```python
from build123d import *

# Parameters (mm, degrees)
SKETCH_1_R      = 5
EXTRUDE_1_DEPTH = 60
SKETCH_2_R      = 3.5
EXTRUDE_2_DEPTH = 2
EXTRUDE_START   = 2
SKETCH_3_R      = 3.5
EXTRUDE_3_DEPTH = 2
EXTRUDE_START_2 = 124
SKETCH_4_R      = 5
EXTRUDE_4_DEPTH = 124
SKETCH_5_R      = 5
EXTRUDE_5_DEPTH = 124
SKETCH_6_R      = 3.5
EXTRUDE_6_DEPTH = 2
SKETCH_7_R      = 5
EXTRUDE_7_DEPTH = 10
SKETCH_8_R      = 3.5
EXTRUDE_8_DEPTH = 2
EXTRUDE_START_3 = 10
SKETCH_9_R      = 5
EXTRUDE_9_DEPTH = 10


with BuildPart() as part:
    # 草图1 → 凸台-拉伸1 (new body)
    with BuildSketch(Plane.XY):
        Circle(SKETCH_1_R)
    extrude(amount=EXTRUDE_1_DEPTH)

    # 草图2 → 凸台-拉伸2 (add)
    with BuildSketch(Plane.XY.offset(60)):
        Circle(SKETCH_2_R)
    extrude(amount=EXTRUDE_2_DEPTH)

    # 草图3 → 凸台-拉伸3 (add)
    with BuildSketch(Plane(origin=(0, 0, 0), x_dir=(-1, 0, 0), z_dir=(0, 0, -1)).offset(EXTRUDE_START)):
        with Locations(Location((0, 0, 0), (0, 0, 180))):
            Circle(SKETCH_3_R)
    extrude(amount=-EXTRUDE_3_DEPTH)

    # 草图4 → 凸台-拉伸4 (add)
    with BuildSketch(Plane(origin=(0, 0, -2), x_dir=(-1, 0, 0), z_dir=(0, 0, -1)).offset(EXTRUDE_START_2)):
        with Locations(Location((0, 0, 0), (0, 0, 180))):
            Circle(SKETCH_4_R)
    extrude(amount=-EXTRUDE_4_DEPTH)

    # 草图5 → 凸台-拉伸5 (add)
    with BuildSketch(Plane.XY.offset(62)):
        Circle(SKETCH_5_R)
    extrude(amount=EXTRUDE_5_DEPTH)

    # 草图6 → 凸台-拉伸6 (add)
    with BuildSketch(Plane.XY.offset(186)):
        Circle(SKETCH_6_R)
    extrude(amount=EXTRUDE_6_DEPTH)

    # 草图7 → 凸台-拉伸7 (add)
    with BuildSketch(Plane.XY.offset(188)):
        Circle(SKETCH_7_R)
    extrude(amount=EXTRUDE_7_DEPTH)

    # 草图8 → 凸台-拉伸8 (add)
    with BuildSketch(Plane(origin=(0, 0, -126), x_dir=(-1, 0, 0), z_dir=(0, 0, -1)).offset(EXTRUDE_START)):
        with Locations(Location((0, 0, 0), (0, 0, 180))):
            Circle(SKETCH_8_R)
    extrude(amount=-EXTRUDE_8_DEPTH)

    # 草图9 → 凸台-拉伸9 (add)
    with BuildSketch(Plane(origin=(0, 0, -128), x_dir=(-1, 0, 0), z_dir=(0, 0, -1)).offset(EXTRUDE_START_3)):
        with Locations(Location((0, 0, 0), (0, 0, 180))):
            Circle(SKETCH_9_R)
    extrude(amount=-EXTRUDE_9_DEPTH)


solid = part.part
```
Source: CAD feature listing. Evaluate the final solid. Frame: model axes, mm. A direction names the side the tool comes from. Round coordinates to 2 decimals unless told otherwise and drop trailing zeros. Loops run counter-clockwise (first coordinate to the right, second up) from the corner with the lowest first, then second, coordinate; pieces in that order, holes last. Notation, with made-up numbers: M 79,80 L 118,80 A25 cw 118,93 Z; hole C 2,58.5 d5. An arc over 180 degrees is marked long. Use a Markdown table: item, result. Add a question column.
1. Contact query for flat-ended pins moving along their axis: P1, Ø4, axis at y = -3.5, z = 2.5, coming from the +X side; P2, Ø1.5, axis at y = -2.5, z = 98.5, coming from the +X side; P3, Ø4, axis at x = 3, z = 87.5, coming from the -Y side. Output: stop coordinate, or through.
2. Line query: line 1 (Z direction, x = 4, y = -1.75); line 2 (Y direction, x = 0.5, z = -9); line 3 (Y direction, x = 1, z = 79.5). Output: solid intervals per line, ascending.
3. Section query A-A on z = 68.5. Return the cut outline in (x, y).
4. Mould query, pull axis Z, two halves, no side actions, for faces 3 (the flat face through (0, 0, -138)), 4 (the cylindrical face through (3.233, -1.341, 60.986)), 5 (the cylindrical face through (-1.08, -4.88, 123.13)). Classes: pulls with the +Z half, pulls with the -Z half, needs draft (parallel to the pull), parting line crosses it, or undercut.
5. Reachability of faces 1 (the cylindrical face through (-5, 0, -133)), 2 (the flat face through (2.2, -3.3, 188)) from +Z, -Z, +X, -X, +Y, -Y: full face, straight path, thin tool, end or side. Return the list, or none.
Reported:
| question | item | result |
|---|---|---|
| 1 | P1 | stops at x = 4.77 |
| 1 | P2 | stops at x = 4.68 |
| 1 | P3 | stops at y = -4.9 |
| 2 | line 1 | z = -138 to -128, -126 to -2, 0 to 60, 62 to 186, 188 to 198 |
| 2 | line 2 | y = -4.97 to 4.97 |
| 2 | line 3 | y = -4.9 to 4.9 |
| 3 | outline | C 0,0 d10 |
| 4 | face 3 | pulls with the -Z half |
| 4 | face 4 | undercut |
| 4 | face 5 | needs draft |
| 5 | face 1 | +Z, -Z |
| 5 | face 2 | none |
